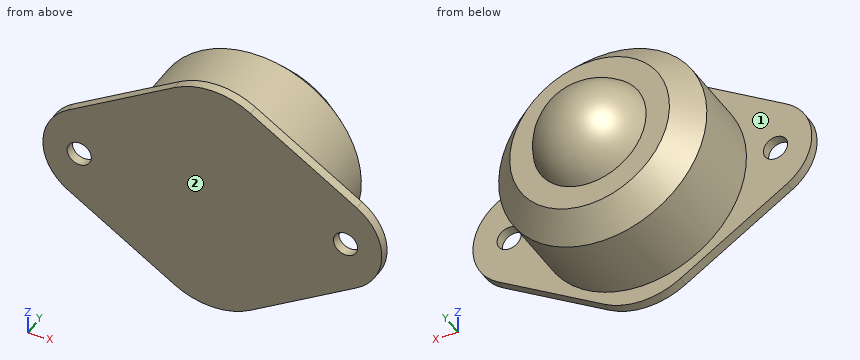
```python
from build123d import *

# Parameters (mm, degrees)
SKETCH_2_R      = 2.5
EXTRUDE_1_DEPTH = 2


with BuildPart() as part:
    # 草图1 → 旋转2 (revolve)
    with BuildSketch(Plane.XY, mode=Mode.PRIVATE) as revolve_2_sk:
        with BuildLine():
            ThreePointArc((0, 12.5), (-7.079662177, 10.301863107), (-11.669393693, 4.480541354))
            Line((-11.669393693, 4.480541354), (-16.5, 4.480541354))
            Line((-16.5, 4.480541354), (-21.5, -0.519458646))
            Line((-21.5, -0.519458646), (-21.5, -15.5))
            Line((-21.5, -15.5), (0, -15.5))
            Line((0, -15.5), (0, 12.5))
        make_face()
    revolve(revolve_2_sk.sketch.rotate(Axis((0, 0, 0), (0, 1, 0)), 270), axis=Axis((0, 0, 0), (0, 1, 0)))

    # 草图2 → 凸台-拉伸1 (add)
    with BuildSketch(Plane.XZ.offset(15.5)):
        with BuildLine():
            Line((-29.841345501, 9.236236767), (-7.866752906, 22.771616919))
            ThreePointArc((-7.866752906, 22.771616919), (0, 25), (7.866752906, 22.771616919))
            Line((7.866752906, 22.771616919), (29.841345501, 9.236236767))
            ThreePointArc((29.841345501, 9.236236767), (35, 0), (29.841345501, -9.236236767))
            Line((29.841345501, -9.236236767), (7.866752906, -22.771616919))
            ThreePointArc((7.866752906, -22.771616919), (0, -25), (-7.866752906, -22.771616919))
            Line((-7.866752906, -22.771616919), (-29.841345501, -9.236236767))
            ThreePointArc((-29.841345501, -9.236236767), (-35, 0), (-29.841345501, 9.236236767))
        make_face()
        with Locations(Location((-27.5, 0, 0), (0, 0, 270))):
            Circle(SKETCH_2_R, mode=Mode.SUBTRACT)
        with Locations(Location((27.5, 0, 0), (0, 0, 90))):
            Circle(SKETCH_2_R, mode=Mode.SUBTRACT)
    extrude(amount=EXTRUDE_1_DEPTH)


solid = part.part
```
The model under review builds one solid part; all positions refer to its coordinate system, in mm. Face numbers are marked on the shaded views. A direction names the side the tool comes from. Round coordinates to 2 decimals unless told otherwise and drop trailing zeros. Write each loop counter-clockwise with the first axis right and the second up, starting at its lowest first coordinate (ties: lowest second). Pieces come first, ordered by that corner, then holes.
(1) Machinability: for the marked faces 1 and 2, which of the approach directions +Z, -Z, +X, -X, +Y, -Y give a long, thin tool a straight path to every point of the face, cutting with its end or side? Answer none if there is none.
(2) Insertion check: pin 1 (10 mm diameter, centred on y = 6.5, z = 12, fed in from -X); pin 2 (2 mm diameter, centred on x = -10, y = -1.5, fed in from +Z); pin 3 (1 mm diameter, centred on y = -9.5, z = 2, fed in from +X); pin 4 (4.5 mm diameter, centred on x = -27.5, z = 0, fed in from -Y). Each pin has a flat end and moves straight along its axis. Give the tip position at first contact, or say it passes through.
(3) We need section C-C on y = 2.25. Give the boundary of the cut face in (x, z).
(4) We need section D-D on y = -13. Give the boundary of the cut face in (x, z), and give its area (3 significant figures).
(5) We need section A-A on z = 0. Give the boundary of the cut face in (x, y).
(6) Wall thickness on L1, parallel to X at y = -16, z = 2; L2, parallel to Y at x = 2, z = -16; L3, parallel to Y at x = 32, z = 2.5: over which ranges is each line inside the solid? List them lowest first.
(7) We need section B-B on x = 0. Give the boundary of the cut face in (y, z), and give its area (3 significant figures).
Findings below:
1. face 1: +Y
1. face 2: +Z, -Z, +X, -X, -Y
2. pin 1: stops at x = -16.24
2. pin 2: stops at z = 19.53
2. pin 3: stops at x = 21.45
2. pin 4: passes through
3. outline: circle Ø37.46 at (0, 0)
4. outline: circle Ø43 at (0, 0)
4. area: 1,450 mm2
5. outline: (-35, -17.5) - (-30, -17.5) - (-30, -15.5) - (-35, -15.5) - close; (-25, -17.5) - (25, -17.5) - (25, -15.5) - (21.5, -15.5) - (21.5, -0.52) - (16.5, 4.48) - (11.67, 4.48) arc R12.5 ccw to (-11.67, 4.48) - (-16.5, 4.48) - (-21.5, -0.52) - (-21.5, -15.5) - (-25, -15.5) - close; (30, -17.5) - (35, -17.5) - (35, -15.5) - (30, -15.5) - close
6. L1: x = -34.81 to -29, -26 to 26, 29 to 34.81
6. L2: y = -17.5 to 4.48
6. L3: y = -17.5 to -15.5
7. outline: (-17.5, -25) - (-15.5, -25) - (-15.5, -21.5) - (-0.52, -21.5) - (4.48, -16.5) - (4.48, -11.67) arc R12.5 ccw to (4.48, 11.67) - (4.48, 16.5) - (-0.52, 21.5) - (-15.5, 21.5) - (-15.5, 25) - (-17.5, 25) - close
7. area: 1,070 mm2
